Design review of the part built by this model. Coordinates are the model's own, in mm. Round coordinates to 2 decimals unless told otherwise and drop trailing zeros. Order: outer loops, then holes, each group sorted by start corner. A loop starts at its lowest first (then second) coordinate and runs counter-clockwise, first axis right, second up. Notation, with made-up numbers: M 76.5,42 L 110.5,42 A23 cw 110.5,62 Z; hole C 39,72.25 d6. An arc over 180 degrees is marked long. Use a Markdown table: item, result. Add a question column.
(1) Take a section at B-B (y = 3.75). Write out the cut boundary in (x, z).
(2) Take a section at A-A (z = 0). Write out the cut boundary in (x, y), then the cut area to 3 significant figures.
(3) For pin 1 (6 mm diameter, centred on y = 7.5, z = 15, fed in from -X); pin 2 (1.5 mm diameter, centred on y = 1.5, z = 42, fed in from -X); pin 3 (9 mm diameter, centred on x = -153.98, z = 88.9, fed in from -Y); pin 4 (3 mm diameter, centred on x = -152.5, y = 2.5, fed in from +Z), all flat-tipped, find the tip position at first contact; note any pin that passes through.
(4) To check wall thickness, follow probe 1 along Z at (x, y) = (0, 6.25); probe 2 along Z at (x, y) = (-2.5, 8.25); probe 3 along X at (y, z) = (7.5, -88.9). State the ranges of each line that lie inside material, in increasing order. Write a range as from..to.
(5) Take a section at C-C (x = 22). Write out the cut boundary in (y, z).
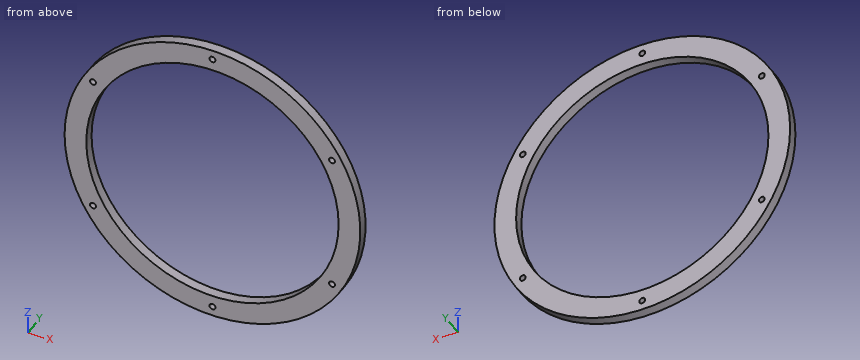
Autodesk Inventor part; units mm, degrees
ref_plane "YZ Plane" through (0, 0, 0) normal (1, 0, 0) x (0, 1, 0)
ref_plane "XZ Plane" through (0, 0, 0) normal (0, 1, 0) x (-1, 0, 0)
ref_plane "XY Plane" through (0, 0, 0) normal (0, 0, 1) x (1, 0, 0)
sketch "Sketch1" plane through (0, 0, 0) normal (0, 1, 0) x (-1, 0, 0)
  circle A0 centre (0, 0) radius 162.56
  circle A1 centre (0, 0) radius 190.5
  dimension "d0" = 325.12
  dimension "d1" = 381
extrude "Extrusion1" add sketch "Sketch1" along normal blind 12.7
sketch "Sketch2" plane through (0, 12.7, 0) normal (0, 1, 0) x (1, 0, 0)
  line L0 (0, 0) -> (0, -177.8) construction
  line L1 (0, 0) -> (177.8, 0) construction
  circle A0 centre (0, -177.8) radius 3.81
  circle A1 centre (153.9793, -88.9) radius 3.81
  circle A2 centre (153.9793, 88.9) radius 3.81
  circle A3 centre (0, 177.8) radius 3.81
  circle A4 centre (-153.9793, 88.9) radius 3.81
  circle A5 centre (-153.9793, -88.9) radius 3.81
  dimension "d6" = 177.8
  dimension "d7" = 90
  dimension "d8" = 7.62
  dimension "d9" = 360
extrude "Extrusion2" cut sketch "Sketch2" against normal through all
properties part number "Turntable Sheath" material "PVC-Piping"
Verdict:
| question | item | result |
|---|---|---|
| 1 | outline | C 0,0 d381; hole C 0,0 d325.12; hole C -153.98,-88.9 d7.62; hole C -153.98,88.9 d7.62; hole C 0,-177.8 d7.62; hole C 0,177.8 d7.62; hole C 153.98,-88.9 d7.62; hole C 153.98,88.9 d7.62 |
| 2 | outline | M -190.5,0 L -162.56,0 L -162.56,12.7 L -190.5,12.7 Z; M 162.56,0 L 190.5,0 L 190.5,12.7 L 162.56,12.7 Z |
| 2 | area | 710 mm^2 |
| 3 | pin 1 | stops at x = -190.12 |
| 3 | pin 2 | stops at x = -185.98 |
| 3 | pin 3 | stops at y = 0 |
| 3 | pin 4 | stops at z = 116.14 |
| 4 | probe 1 | z = -190.5..-181.61, -173.99..-162.56, 162.56..173.99, 181.61..190.5 |
| 4 | probe 2 | z = -190.48..-180.68, -174.92..-162.54, 162.54..174.92, 180.68..190.48 |
| 4 | probe 3 | x = -168.48..-157.79, -150.17..-136.1, 136.1..150.17, 157.79..168.48 |
| 5 | outline | M 0,-189.23 L 12.7,-189.23 L 12.7,-161.06 L 0,-161.06 Z; M 0,161.06 L 12.7,161.06 L 12.7,189.23 L 0,189.23 Z |
